from build123d import *

# Parameters (mm, degrees)
F0_R     = 1.905
F0_R_2   = 4.0005
F0_R_3   = 2.3495
F1_DEPTH = 6.35


with BuildPart() as f1:
    # F0 (on Top) → F1 (new body)
    with BuildSketch(Plane.XY):
        with BuildLine():
            ThreePointArc((0, 6.35), (-1.859872, 10.840128), (-6.35, 12.7))
            Line((-6.35, 12.7), (-88.9, 12.7))
            Line((-88.9, 12.7), (-90.216626, 12.7))
            ThreePointArc((-90.216626, 12.7), (-120.90146, 6.35), (-90.216626, 0))
            Line((-90.216626, 0), (-88.9, 0))
            Line((-88.9, 0), (-6.35, 0))
            ThreePointArc((-6.35, 0), (-1.859872, 1.859872), (0, 6.35))
        make_face()
        with Locations((-104.902, -1.651)):
            Circle(F0_R, mode=Mode.SUBTRACT)
        with Locations((-112.903, 6.35)):
            Circle(F0_R, mode=Mode.SUBTRACT)
        with Locations((-104.902, 6.35)):
            Circle(F0_R_2, mode=Mode.SUBTRACT)
        with Locations((-96.901, 6.35)):
            Circle(F0_R, mode=Mode.SUBTRACT)
        with Locations((-104.902, 14.351)):
            Circle(F0_R, mode=Mode.SUBTRACT)
        with Locations((-6.35, 6.35)):
            Circle(F0_R_3, mode=Mode.SUBTRACT)
    extrude(amount=F1_DEPTH)


solid = f1.part
Input: part model. Units: mm. Frame: model coordinates. A direction names the side the tool comes from. Give positions to 0.01 mm unless a question says otherwise; leave off trailing zeros. Order: outer loops, then holes, each group sorted by start corner. A loop starts at its lowest first (then second) coordinate and runs counter-clockwise, first axis right, second up. Notation, with made-up numbers: M 9,55.5 L 63,55.5 A23 ccw 63,66.5 Z; hole C -22.5,69.5 d3. An arc over 180 degrees is marked long. Answer as a JSON object with one key per item and string values.
1. First-contact query: P1, Ø2.5, axis at x = -112.903, y = 6.35, coming from the +Z side; P2, Ø2, axis at y = 2.5, z = 5, coming from the -X side; P3, Ø1.9, axis at x = -40.5, z = 3, coming from the -Y side; P4, Ø1.5, axis at x = -91.5, z = 4.5, coming from the -Y side. Flat tips, straight axial feed; report the tip coordinate or a pass-through.
Result sheet:
{"P1": "through", "P2": "x = -120.65", "P3": "y = 0", "P4": "y = -3.44"}
2. Cut plane B-B, the plane x = -14.5. Output: boundary loops of the cut face in (y, z).
Result sheet:
{"outline": "M 0,0 L 12.7,0 L 12.7,6.35 L 0,6.35 Z"}
3. Pull-direction query (Y, two-part tool) for faces 1 (the cylindrical face through (-111.143, 5.62, 3.131)), 2 (the flat face through (-49, 0, 3)), 3 (the flat face through (-75, 7, 6.35)); classes: +Y half, -Y half, draft (parallel to the pull), parting line (faces both ways), or undercut.
Result sheet:
{"face 1": "undercut", "face 2": "-Y half", "face 3": "draft"}
4. Ray query, line 1 (Y direction, x = -6.35, z = 2.75); line 2 (Y direction, x = -57.5, z = 3.25); line 3 (X direction, y = -2.5, z = 2). Return the intervals inside material, ascending. Write a range as [from, to].
Result sheet:
{"line 1": "[0, 4], [8.7, 12.7]", "line 2": "[0, 12.7]", "line 3": "[-118.23, -106.61], [-103.2, -91.57]"}
5. Cut plane A-A, the plane z = 4.5. State how many separate pieces and enclosed holes the cut face has, and give its area (3 significant figures).
Result sheet:
{"separate pieces": "1", "enclosed holes": "6", "area": "1,810 mm²"}
6. Reachability of faces 4 (the flat face through (-48, 12.7, 3)), 5 (the flat face through (-75, 7, 0)) from +Z, -Z, +X, -X, +Y, -Y: full face, straight path, thin tool, end or side. Return the list, or none.
Result sheet:
{"face 4": "+Z, -Z, +X, +Y", "face 5": "-Z, +X, -X, +Y, -Y"}
